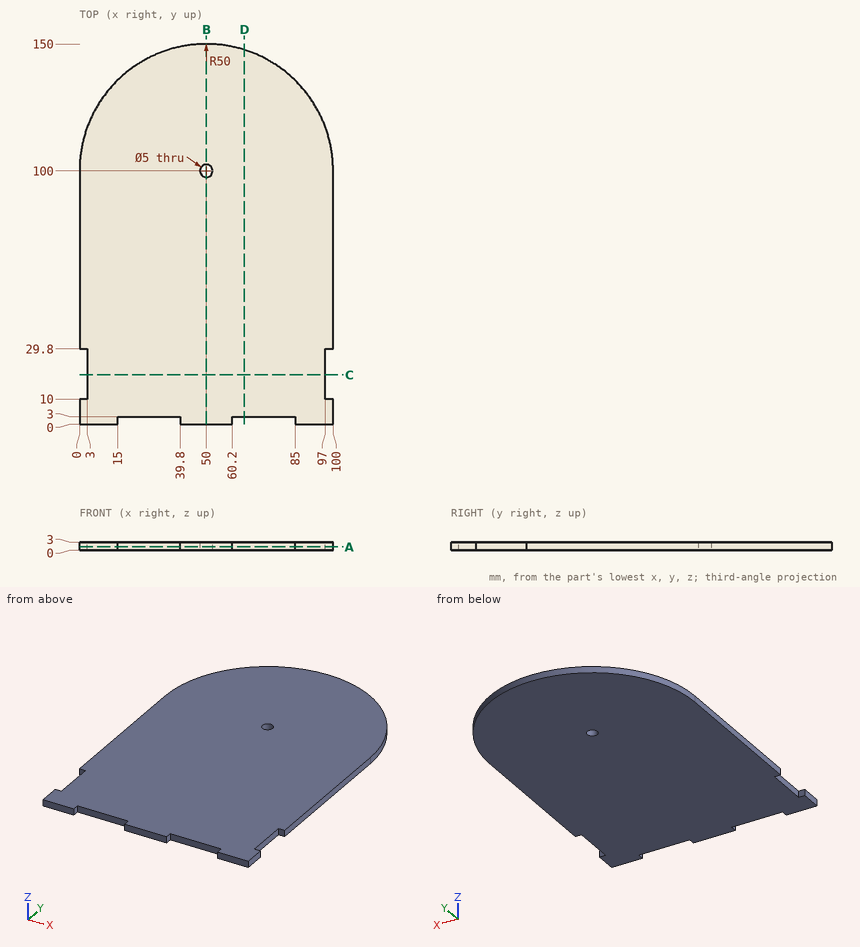
Could you check a few things on this drawing? It's one solid part, dimensions in mm from its lowest x, y, z. Coordinates: 2 decimals unless noted, no trailing zeros. Order: outer loops, then holes, each group sorted by start corner. A loop starts at its lowest first (then second) coordinate and runs counter-clockwise, first axis right, second up. Notation, with made-up numbers: (46, 54) -> (104, 54) arc R20 ccw to (104, 67) -> close; hole circle Ø3 at (-31.5, 9.5). An arc over 180 degrees is marked (long way). One line per item, written item: value. Start each with the question number.
1) I'm going to push flat-ended pins straight in: pin 1 (0.9 mm diameter, centred on x = 98.5, z = 1.5, fed in from -Y); pin 2 (3 mm diameter, centred on x = 50, y = 100, fed in from +Z); pin 3 (1.5 mm diameter, centred on x = 76, z = 1, fed in from -Y); pin 4 (0.9 mm diameter, centred on y = 24.5, z = 1.5, fed in from -X). Where does each tip first touch, or does it pass through?
2) Imagine slicing it at D-D on x = 65. List the corners of the cut face in (y, z) for me.
3) If I drill on L1, parallel to Y at x = 50, z = 1.05; L2, parallel to X at y = 27, z = 1.75; L3, parallel to X at y = 121.5, z = 1.65, over which ranges is the centre line in solid material (lowest first)? Write a range as [from, to].
4) Imagine slicing it at C-C on y = 19.5. List the corners of the cut face in (x, z) for me.
5) Imagine slicing it at B-B on x = 50. List the corners of the cut face in (y, z) for me, plus the area to 3 significant figures.
6) Imagine slicing it at A-A on z = 1.25. List the corners of the cut face in (x, y) for me.
Answer list:
1. pin 1: stops at y = 0
1. pin 2: passes through
1. pin 3: stops at y = 3
1. pin 4: stops at x = 3
2. outline: (3, 0) -> (147.7, 0) -> (147.7, 3) -> (3, 3) -> close
3. L1: y = [0, 97.5], [102.5, 150]
3. L2: x = [3, 97]
3. L3: x = [4.86, 95.14]
4. outline: (3, 0) -> (97, 0) -> (97, 3) -> (3, 3) -> close
5. outline: (0, 0) -> (97.5, 0) -> (97.5, 3) -> (0, 3) -> close; (102.5, 0) -> (150, 0) -> (150, 3) -> (102.5, 3) -> close
5. area: 435 mm2
6. outline: (0, 0) -> (15, 0) -> (15, 3) -> (39.8, 3) -> (39.8, 0) -> (60.2, 0) -> (60.2, 3) -> (85, 3) -> (85, 0) -> (100, 0) -> (100, 10) -> (97, 10) -> (97, 29.8) -> (100, 29.8) -> (100, 100) arc R50 ccw to (0, 100) -> (0, 29.8) -> (3, 29.8) -> (3, 10) -> (0, 10) -> close; hole circle Ø5 at (50, 100)
